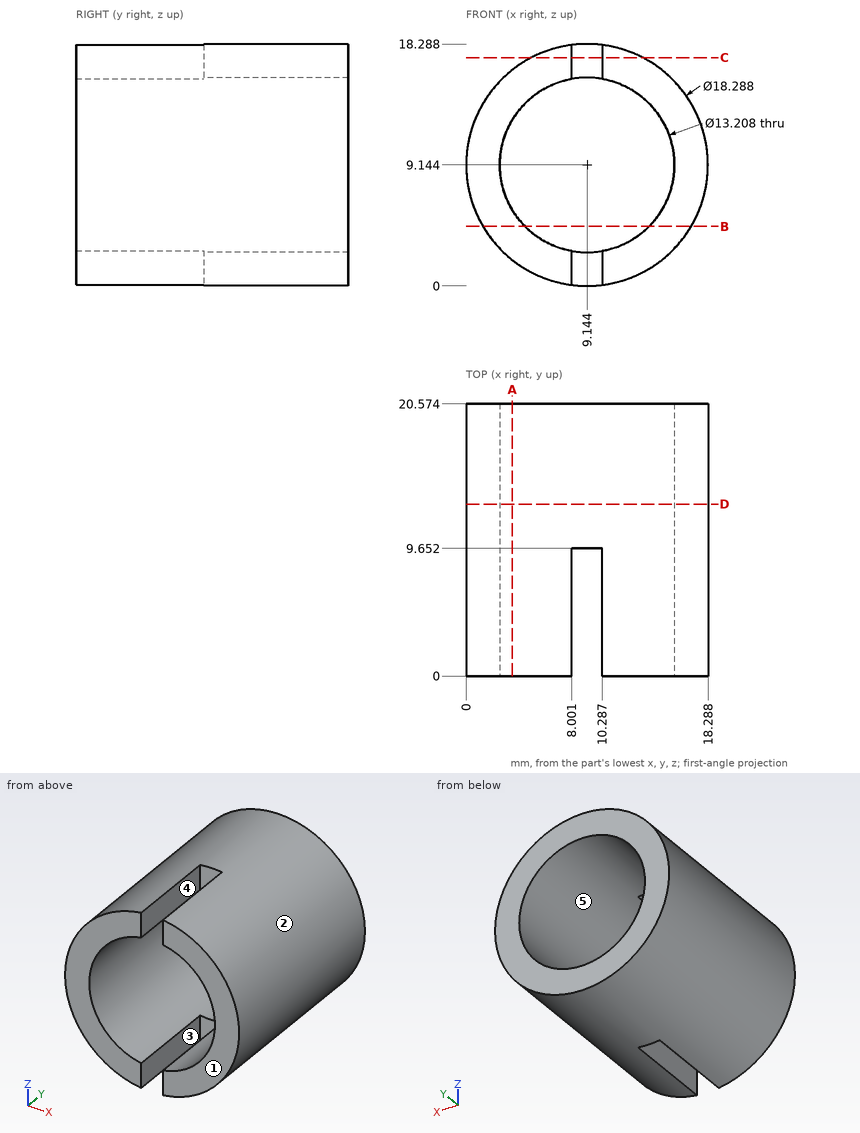
Design review of the part shown in the three views and the two pictorial views. Dimensions are in mm from the part's minimum x, y and z. A direction names the side the tool comes from. Coordinates: 2 decimals unless noted, no trailing zeros. Write each loop counter-clockwise with the first axis right and the second up, starting at its lowest first coordinate (ties: lowest second). Pieces come first, ordered by that corner, then holes.
(1) Add section C-C on z = 17.25. Give the boundary of the cut face in (x, y).
(2) Tool access review of the marked faces 4 and 5: name each direction out of +Z, -Z, +X, -X, +Y, -Y from which nothing blocks a thin tool from reaching the whole face with its end or side.
(3) For pin 1 Ø1.3 at (y, z) = (3.5, 17) entering from -X; pin 2 Ø1.3 at (y, z) = (6.5, 2) entering from -X; pin 3 Ø5 at (x, y) = (12, 17) entering from +Z, all flat-tipped, find the tip position at first contact; note any pin that passes through.
(4) Add section A-A on x = 3.5. Give the boundary of the cut face in (y, z) (3 decimals), then the cut area to 3 significant figures.
(5) Add section D-D on y = 13. Give the boundary of the cut face in (x, z).
(6) The part is to be moulded in two halves that separate along X. For the marked faces 1, 2 and 3, say which applies: +X half, -X half, draft (parallel to the pull), parting line (faces both ways), or undercut.
(7) Wall thickness on probe 1 along X at (y, z) = (8, 17); probe 2 along X at (y, z) = (2.5, 9.5); probe 3 along Z at (x, y) = (13.5, 10.25): over which ranges is each line inside the solid? List them lowest first.
(8) Add section B-B on z = 4.5. Give the boundary of the cut face in (x, y).
Answer sheet:
1. outline: (4.91, 0) - (8, 0) - (8, 9.65) - (10.29, 9.65) - (10.29, 0) - (13.38, 0) - (13.38, 20.57) - (4.91, 20.57) - close
2. face 4: +Z, -Z, -Y
2. face 5: +Y, -Y
3. pin 1: stops at x = 3.51
3. pin 2: stops at x = 2.71
3. pin 3: stops at z = 18.28
4. outline: (0, 1.95) - (20.574, 1.95) - (20.574, 5.715) - (0, 5.715) - close; (0, 12.573) - (20.574, 12.573) - (20.574, 16.338) - (0, 16.338) - close
4. area: 155 mm2
5. outline: circle Ø18.29 at (9.14, 9.14); hole circle Ø13.21 at (9.14, 9.14)
6. face 1: draft
6. face 2: parting line
6. face 3: undercut
7. probe 1: x = 4.46 to 8, 10.29 to 13.82
7. probe 2: x = 0.01 to 2.55, 15.74 to 18.28
7. probe 3: z = 1.1 to 4.18, 14.11 to 17.18
8. outline: (1.27, 0) - (4.45, 0) - (4.45, 20.57) - (1.27, 20.57) - close; (13.84, 0) - (17.02, 0) - (17.02, 20.57) - (13.84, 20.57) - close
